```python
from build123d import *

# Parameters (mm, degrees)
F0_W     = 38.1
F0_H     = 38.1
F1_DEPTH = 295.91
F2_W     = 31.75
F2_H     = 31.75
F3_DEPTH = 25.4
F4_W     = 31.75
F4_H     = 31.75
F5_DEPTH = 25.4
F6_R     = 6.35


with BuildPart() as f1:
    # F0 (on Front) → F1 (new body, symmetric)
    with BuildSketch(Plane.XZ):
        Rectangle(F0_W, F0_H)
    extrude(amount=F1_DEPTH, both=True)

    # F2 (on face) → F3 (join)
    with BuildSketch(Plane(origin=(0, 295.91, 0), x_dir=(-1, 0, 0), z_dir=(0, 1, 0))):
        Rectangle(F2_W, F2_H)
    extrude(amount=F3_DEPTH)

    # F4 (on face) → F5 (join)
    with BuildSketch(Plane.XZ.offset(295.91)):
        Rectangle(F4_W, F4_H)
    extrude(amount=F5_DEPTH)

    # F6
    f6_edges = [f1.edges().sort_by_distance(p)[0] for p in [
        (19.05, 0, 19.05),
        (19.05, 0, -19.05),
        (-19.05, 0, -19.05),
        (-19.05, 0, 19.05),
    ]]
    fillet(f6_edges, radius=F6_R)


solid = f1.part
```
For this review, take the finished solid that the model builds, in its own axes (mm). A direction names the side the tool comes from. Round coordinates to 2 decimals unless told otherwise and drop trailing zeros. Write each loop counter-clockwise with the first axis right and the second up, starting at its lowest first coordinate (ties: lowest second). Pieces come first, ordered by that corner, then holes. Notation, with made-up numbers: (55, 1) -> (114, 1) arc R20 cw to (114, 22) -> close; hole circle Ø2 at (-10, 1.25). An arc over 180 degrees is marked (long way). Use one line per item in the form item = value.
Q1. Machinability: for faces 1 (the flat face through (0, 308, 15.875)), 2 (the flat face through (0, 308, -15.875)), 3 (the flat face through (0, -308, -15.875)), which of the approach directions +Z, -Z, +X, -X, +Y, -Y give a long, thin tool a straight path to every point of the face, cutting with its end or side? Answer none if there is none.
Resolved:
face_1 = +Z, +X, -X, +Y
face_2 = -Z, +X, -X, +Y
face_3 = -Z, +X, -X, -Y
Q2. Clearance check with flat-ended pins moving along their axes: pin 1 Ø20.5 at (y, z) = (-314.5, -5.5) entering from -X (3 decimals); pin 2 Ø20.5 at (y, z) = (-313.5, -2.5) entering from +X (3 decimals); pin 3 Ø7.5 at (x, y) = (-4.5, -304.5) entering from +Z (3 decimals). State where each tip first meets the part, or that it passes through.
Resolved:
pin_1 = -15.875
pin_2 = 15.875
pin_3 = 15.875
Q3. To check wall thickness, follow probe 1 along Y at (x, z) = (13, -16); probe 2 along Z at (x, y) = (-13, -4); probe 3 along Z at (x, y) = (-15.5, -26). State the ranges of each line that lie inside material, in increasing order. Write a range as from..to.
Resolved:
probe_1 = -295.91..295.91
probe_2 = -19.04..19.04
probe_3 = -18.4..18.4
Q4. Consider section A-A (y = 245.5). State the section outline as (x, z) points, then the cut area to 3 significant figures.
Resolved:
outline = (-19.05, -12.7) arc R6.35 ccw to (-12.7, -19.05) -> (12.7, -19.05) arc R6.35 ccw to (19.05, -12.7) -> (19.05, 12.7) arc R6.35 ccw to (12.7, 19.05) -> (-12.7, 19.05) arc R6.35 ccw to (-19.05, 12.7) -> close
area = 1,420 mm²
